Geometry check sheet. Reference: the model listing, model coordinates, mm. A direction names the side the tool comes from. Give positions to 0.01 mm unless a question says otherwise; leave off trailing zeros. Write each loop counter-clockwise with the first axis right and the second up, starting at its lowest first coordinate (ties: lowest second). Pieces come first, ordered by that corner, then holes. Notation, with made-up numbers: (-22, 60.25) -> (-13, 60.25) arc R14 cw to (-13, 68.25) -> close; hole circle Ø6 at (33.5, -31.5). An arc over 180 degrees is marked (long way). Write item = value, one per line. Start each with the question number.
1. Set-up check for faces 5 (the flat face through (7, 2.5, 65)), 6 (the cylindrical face through (-0.5, -2.4, 31.6)), 7 (the flat face through (-7, 2.5, 65)), 8 (the flat face through (10.75, 0, 66)): record each of +Z, -Z, +X, -X, +Y, -Y from which the full face is reachable in a straight line by a thin tool's end or side.
2. Depth check by flat-ended pin: P1, Ø3.5, axis at y = 7, z = 65, coming from the +X side; P2, Ø8, axis at x = 3, z = 49, coming from the +Y side; P3, Ø0.9, axis at x = 5, z = 65.5, coming from the +Y side. Enter the tip coordinate at first touch or a pass-through.
3. Cross-section at C-C, the plane z = 50. Record the cut outline in (x, y), plus the area to 3 significant figures.
4. Mould release check, pull along X, two halves, no side actions. Record for faces 1 (the flat face through (-2, 6, 66)), 2 (the flat face through (11, 0, 67)), 3 (the flat face through (10, 0, 65)), 4 (the flat face through (2, 6, 66)): pulls with the +X half, pulls with the -X half, needs draft (parallel to the pull), parting line crosses it, or undercut.
5. Cross-section at D-D, the plane x = -6.25. Record the cut outline in (y, z), plus the area to 3 significant figures.
6. Cross-section at A-A, the plane x = 0. Record the cut outline in (y, z).
7. Thickness scan on line 1 along Y through (x, z) = (0.25, 49); line 2 along Z through (x, y) = (-7.75, 0); line 3 along Z through (x, y) = (10.5, 0). Record the ranges inside material, lowest first.
8. Cross-section at B-B, the plane y = 0. Record the cut outline in (x, z), plus the area to 3 significant figures.
```python
from build123d import *

# Parameters (mm, degrees)
SKETCH1_R           = 2.45
BOSS_EXTRUDE1_DEPTH = 64
SKETCH2_W           = 24
SKETCH2_H           = 5
BOSS_EXTRUDE2_DEPTH = 3
SKETCH3_W           = 2
SKETCH3_H           = 5
CUT_EXTRUDE2_DEPTH  = 2
SKETCH4_W           = 4
SKETCH4_H           = 8
BOSS_EXTRUDE3_DEPTH = 3
CUT_EXTRUDE3_REACH  = 71.248


with BuildPart() as part:
    # Sketch1 → Boss-Extrude1 (new body)
    with BuildSketch(Plane.XY):
        Circle(SKETCH1_R)
    extrude(amount=BOSS_EXTRUDE1_DEPTH)

    # Sketch2 → Boss-Extrude2 (add)
    with BuildSketch(Plane.XY.offset(64)):
        Rectangle(SKETCH2_W, SKETCH2_H)
    extrude(amount=BOSS_EXTRUDE2_DEPTH)

    # Sketch3 → Cut-Extrude2 (cut)
    with BuildSketch(Plane.XY.offset(67)):
        with Locations((9.75, 0)):
            Rectangle(SKETCH3_W, SKETCH3_H)
        with Locations((-9.75, 0)):
            Rectangle(SKETCH3_W, SKETCH3_H)
    extrude(amount=-CUT_EXTRUDE2_DEPTH, mode=Mode.SUBTRACT)

    # Sketch4 → Boss-Extrude3 (add)
    with BuildSketch(Plane.XY.offset(67)):
        with Locations((0, 6.5)):
            Rectangle(SKETCH4_W, SKETCH4_H)
    extrude(amount=-BOSS_EXTRUDE3_DEPTH)

    # Sketch5 → Cut-Extrude3 (cut, up to next)
    with BuildSketch(Plane(origin=(2, 0, 0), x_dir=(0, 0, -1), z_dir=(1, 0, 0)), mode=Mode.PRIVATE) as cut_extrude3_sk1:
        Polygon((-67, 10.5), (-64, 7.9), (-64, 10.5), align=None)
    cut_extrude3_tool1 = extrude(cut_extrude3_sk1.sketch, amount=-CUT_EXTRUDE3_REACH, mode=Mode.PRIVATE) & part.part
    add(cut_extrude3_tool1.solids().sort_by_distance((2, 9.633333, 65))[0], mode=Mode.SUBTRACT)


solid = part.part
```
Answers:
q1.face_5 = +Z, -Z, +X, +Y
q1.face_6 = -Z
q1.face_7 = +Z, -Z, -X, +Y
q1.face_8 = +Z, +Y, -Y
q2.P1 = 2
q2.P2 = 2.45
q2.P3 = 2.5
q3.outline = circle Ø4.9 at (0, 0)
q3.area = 18.9 mm^2
q4.face_1 = pulls with the -X half
q4.face_2 = needs draft
q4.face_3 = undercut
q4.face_4 = pulls with the +X half
q5.outline = (-2.5, 64) -> (2.5, 64) -> (2.5, 67) -> (-2.5, 67) -> close
q5.area = 15.0 mm^2
q6.outline = (-2.5, 64) -> (-2.45, 64) -> (-2.45, 0) -> (2.45, 0) -> (2.45, 64) -> (7.9, 64) -> (10.5, 67) -> (-2.5, 67) -> close
q7.line_1 = -2.44 to 2.44
q7.line_2 = 64 to 67
q7.line_3 = 64 to 65
q8.outline = (-12, 64) -> (-2.45, 64) -> (-2.45, 0) -> (2.45, 0) -> (2.45, 64) -> (12, 64) -> (12, 67) -> (10.75, 67) -> (10.75, 65) -> (8.75, 65) -> (8.75, 67) -> (-8.75, 67) -> (-8.75, 65) -> (-10.75, 65) -> (-10.75, 67) -> (-12, 67) -> close
q8.area = 378 mm^2
